Here's the drawing with two shaded views (mm, measured from the low corner). I have some questions. A direction names the side the tool comes from. Round coordinates to 2 decimals unless told otherwise and drop trailing zeros. Order: outer loops, then holes, each group sorted by start corner. A loop starts at its lowest first (then second) coordinate and runs counter-clockwise, first axis right, second up.
Q1. We'd pull the mould along X, two halves only. Please class the marked faces 1 and 2: pulls with the +X half, pulls with the -X half, needs draft (parallel to the pull), parting line crosses it, or undercut.
Q2. If I drill on line 1 (Y direction, x = 29, z = 3.25); line 2 (Y direction, x = 29, z = 7); line 3 (X direction, y = 83, z = 7.25), over which ranges is the centre line in solid material (lowest first)?
Q3. For the marked faces 3, 4 and 5, which set-ups out of +Z, -Z, +X, -X, +Y, -Y let a thin tool reach every point of the face, with its end or its side?
Q4. Will these pins go through, and if not, where does the flat tip stop? P1, Ø1, axis at x = 52.5, y = 18.5, coming from the +Z side; P2, Ø9, axis at x = 43, y = 30.5, coming from the -Z side; P3, Ø2.5, axis at y = 56.5, z = 7.5, coming from the -X side.
Q5. If we section it at B-B (y = 41): Please give me the cut outline in (x, z).
Q6. If we section it at A-A (x = 51.5): Please give me the cut outline in (y, z), plus the area to 4 significant figures.
Q7. If we section it at C-C (x = 71): Please give me the cut outline in (y, z).
Q8. If we section it at D-D (y = 11): Please give me the cut outline in (x, z), plus the area to 3 significant figures.
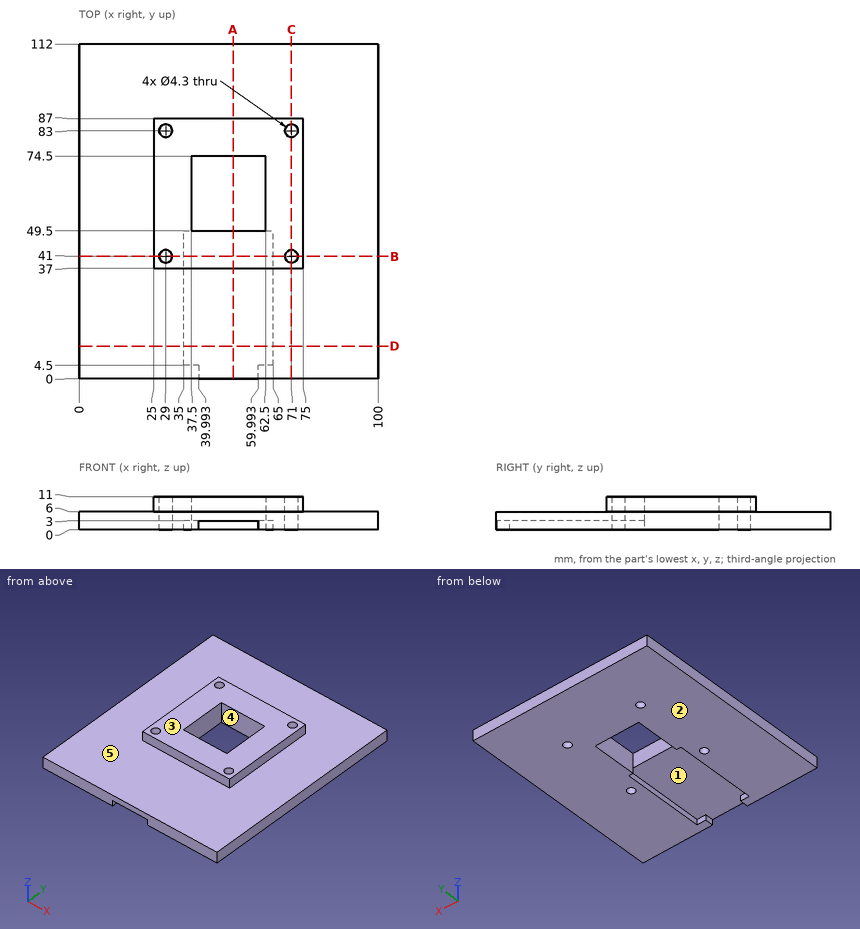
Solution:
1. face 1: undercut
1. face 2: needs draft
2. line 1: y = 0 to 38.85, 43.15 to 80.85, 85.15 to 112
2. line 2: y = 37 to 38.85, 43.15 to 80.85, 85.15 to 87
2. line 3: x = 25 to 26.85, 31.15 to 68.85, 73.15 to 75
3. face 3: +Z, +X, -X, +Y, -Y
3. face 4: +Z, -Z
3. face 5: +Z
4. P1: stops at z = 6
4. P2: stops at z = 3
4. P3: stops at x = 25
5. outline: (0, 0) - (26.85, 0) - (26.85, 11) - (25, 11) - (25, 6) - (0, 6) - close; (31.15, 0) - (35, 0) - (35, 3) - (65, 3) - (65, 0) - (68.85, 0) - (68.85, 11) - (31.15, 11) - close; (73.15, 0) - (100, 0) - (100, 6) - (75, 6) - (75, 11) - (73.15, 11) - close
6. outline: (0, 3) - (49.5, 3) - (49.5, 11) - (37, 11) - (37, 6) - (0, 6) - close; (74.5, 0) - (112, 0) - (112, 6) - (87, 6) - (87, 11) - (74.5, 11) - close
6. area: 498.5 mm2
7. outline: (0, 0) - (38.85, 0) - (38.85, 11) - (37, 11) - (37, 6) - (0, 6) - close; (43.15, 0) - (80.85, 0) - (80.85, 11) - (43.15, 11) - close; (85.15, 0) - (112, 0) - (112, 6) - (87, 6) - (87, 11) - (85.15, 11) - close
8. outline: (0, 0) - (35, 0) - (35, 3) - (65, 3) - (65, 0) - (100, 0) - (100, 6) - (0, 6) - close
8. area: 510 mm2
